```python
from build123d import *

# Parameters (mm, degrees)
SKETCH1_R              = 19
BOSS_EXTRUDE1_DEPTH    = 24
SKETCH2_R              = 13
CUT_EXTRUDE1_DEPTH     = 8
SKETCH3_R              = 6
CUT_EXTRUDE2_DEPTH     = 32.272991542
SKETCH4_R              = 12.5
CUT_EXTRUDE3_DEPTH     = 8
SKETCH5_W              = 22
SKETCH5_H              = 22
CUT_EXTRUDE4_DEPTH     = 8
CUT_EXTRUDE5_START     = 12
CUT_EXTRUDE5_OUTLINE_R = 6
CUT_EXTRUDE5_DEPTH     = 7.000000101
SKETCH6_R              = 1.5
CUT_EXTRUDE6_DEPTH     = 32.272991715
SKETCH7_R              = 1.5
CUT_EXTRUDE7_DEPTH     = 24


# Read off the part's stored shape, not the designer's step: Cut-Extrude5
with BuildPart() as part:
    # Sketch1 → Boss-Extrude1 (new body)
    with BuildSketch(Plane(origin=(0, 0, 0), x_dir=(1, 0, 0), z_dir=(0, 1, 0))):
        with Locations(Location((0, 0, 0), (0, 0, 270))):
            Circle(SKETCH1_R)
    extrude(amount=BOSS_EXTRUDE1_DEPTH)

    # Sketch2 → Cut-Extrude1 (cut)
    with BuildSketch(Plane(origin=(0, 24, 0), x_dir=(1, 0, 0), z_dir=(0, 1, 0))):
        with Locations(Location((0, 0, 0), (0, 0, 270))):
            Circle(SKETCH2_R)
    extrude(amount=-CUT_EXTRUDE1_DEPTH, mode=Mode.SUBTRACT)

    # Sketch3 → Cut-Extrude2 (cut, through all)
    with BuildSketch(Plane(origin=(0, 16, 0), x_dir=(1, 0, 0), z_dir=(0, 1, 0))):
        with Locations(Location((0, 0, 0), (0, 0, 270))):
            Circle(SKETCH3_R)
    extrude(amount=-CUT_EXTRUDE2_DEPTH, mode=Mode.SUBTRACT)

    # Sketch4 → Cut-Extrude3 (cut)
    with BuildSketch(Plane.XZ):
        with Locations(Location((0, 0, 0), (0, 0, 270))):
            Circle(SKETCH4_R)
    extrude(amount=-CUT_EXTRUDE3_DEPTH, mode=Mode.SUBTRACT)

    # Sketch5 → Cut-Extrude4 (cut)
    with BuildSketch(Plane.XZ):
        Rectangle(SKETCH5_W, SKETCH5_H)
    extrude(amount=-CUT_EXTRUDE4_DEPTH, mode=Mode.SUBTRACT)

    # Cut-Extrude5 outline → Cut-Extrude5 (cut)
    with BuildSketch(Plane.XY.offset(CUT_EXTRUDE5_START)):
        with Locations((-0.045844334, 12)):
            Circle(CUT_EXTRUDE5_OUTLINE_R)
    extrude(amount=CUT_EXTRUDE5_DEPTH, mode=Mode.SUBTRACT)

    # Sketch6 → Cut-Extrude6 (cut, through all)
    with BuildSketch(Plane(origin=(0, 16, 0), x_dir=(1, 0, 0), z_dir=(0, 1, 0))):
        with Locations(Location((-6.01040764, 6.01040764, 0), (0, 0, 270))):
            Circle(SKETCH6_R)
        with Locations(Location((6.01040764, -6.01040764, 0), (0, 0, 270))):
            Circle(SKETCH6_R)
    extrude(amount=-CUT_EXTRUDE6_DEPTH, mode=Mode.SUBTRACT)

    # Sketch7 → Cut-Extrude7 (cut)
    with BuildSketch(Plane(origin=(0, 24, 0), x_dir=(1, 0, 0), z_dir=(0, 1, 0))):
        with Locations(Location((11.313708499, -11.313708499, 0), (0, 0, 270))):
            Circle(SKETCH7_R)
        with Locations(Location((-11.313708499, -11.313708499, 0), (0, 0, 270))):
            Circle(SKETCH7_R)
        with Locations(Location((-11.313708499, 11.313708499, 0), (0, 0, 270))):
            Circle(SKETCH7_R)
        with Locations(Location((11.313708499, 11.313708499, 0), (0, 0, 270))):
            Circle(SKETCH7_R)
    extrude(amount=-CUT_EXTRUDE7_DEPTH, mode=Mode.SUBTRACT)


solid = part.part
```
Design review of the part built by this model. Coordinates are the model's own, in mm. A direction names the side the tool comes from. Round coordinates to 2 decimals unless told otherwise and drop trailing zeros. Order: outer loops, then holes, each group sorted by start corner. A loop starts at its lowest first (then second) coordinate and runs counter-clockwise, first axis right, second up. Notation, with made-up numbers: (-14.5, -3.75) - (11.5, -3.75) arc R15 cw to (11.5, 11.25) - close; hole circle Ø11 at (-38.75, -37). An arc over 180 degrees is marked (long way). Return JSON: item names as keys, results as strings.
Q1. Consider section B-B on z = 0. Write out the cut boundary in (x, y).
Computed values:
{"outline": "(-19, 0) - (-12.5, 0) - (-12.5, 8) - (-6, 8) - (-6, 16) - (-13, 16) - (-13, 24) - (-19, 24) - close; (6, 8) - (12.5, 8) - (12.5, 0) - (19, 0) - (19, 24) - (13, 24) - (13, 16) - (6, 16) - close"}
Q2. The part is to be moulded in two halves that separate along X. For faces 1 (the cylindrical face through (5.436, 12.056, 7.396)), 2 (the flat face through (-12.4, 0, 4)), 3 (the cylindrical face through (-11.56, 11.83, -15.08)), 4 (the cylindrical face through (12.58, 12.17, 12.12)), say which applies: pulls with the +X half, pulls with the -X half, needs draft (parallel to the pull), parting line crosses it, or undercut.
Computed values:
{"face 1": "undercut", "face 2": "needs draft", "face 3": "parting line crosses it", "face 4": "undercut"}
Q3. Machinability: for faces 5 (the flat face through (0, 12, 12)), 6 (the flat face through (8, 4, 11)), 7 (the flat face through (0.2, 16, -6.2)), which of the approach directions +Z, -Z, +X, -X, +Y, -Y give a long, thin tool a straight path to every point of the face, cutting with its end or side? Answer none if there is none.
Computed values:
{"face 5": "+Z", "face 6": "-Y", "face 7": "+Y"}
Q4. Consider section C-C on x = 1.5. Write out the cut boundary in (y, z), plus the area to 3 significant figures.
Computed values:
{"outline": "(0, -18.94) - (24, -18.94) - (24, -12.91) - (16, -12.91) - (16, -5.81) - (8, -5.81) - (8, -12.41) - (0, -12.41) - close; (0, 12.41) - (6.2, 12.41) - (6.2, 18.94) - (0, 18.94) - close; (8, 5.81) - (16, 5.81) - (16, 12) - (8, 12) - close; (17.8, 12.91) - (24, 12.91) - (24, 18.94) - (17.8, 18.94) - close", "area": "333 mm2"}
Q5. Wall thickness on L1, parallel to X at y = 20.5, z = -10; L2, parallel to X at y = 20, z = 0; L3, parallel to X at y = 10.25, z = -12.5: over which ranges is each line inside the solid? List them lowest first. Write a range as [from, to].
Computed values:
{"L1": "x = [-16.16, -12.04], [-10.59, -8.31], [8.31, 10.59], [12.04, 16.16]", "L2": "x = [-19, -13], [13, 19]", "L3": "x = [-14.31, -12.23], [-10.4, 10.4], [12.23, 14.31]"}
Q6. Consider section D-D on x = 7. Write out the cut boundary in (y, z), plus the area to 3 significant figures.
Computed values:
{"outline": "(0, -17.66) - (24, -17.66) - (24, -10.95) - (16, -10.95) - (16, 4.88) - (8, 4.88) - (8, -11) - (0, -11) - close; (0, 11) - (8, 11) - (8, 7.14) - (16, 7.14) - (16, 10.95) - (24, 10.95) - (24, 17.66) - (0, 17.66) - close", "area": "479 mm2"}
Q7. For pin 1 Ø1.2 at (y, z) = (4.5, -7) entering from +X; pin 2 Ø2.5 at (x, y) = (-0.5, 12) entering from +Z; pin 3 Ø1 at (x, y) = (-13.5, 19.5) entering from -Z, all flat-tipped, find the tip position at first contact; note any pin that passes through.
Computed values:
{"pin 1": "stops at x = 17.89", "pin 2": "stops at z = 12", "pin 3": "stops at z = -13.86"}
Q8. Consider section A-A on y = 1.75. Write out the cut boundary in (x, z), plus the area to 3 significant figures.
Computed values:
{"outline": "circle Ø38 at (0, 0); hole (-11, -9.85) arc R1.5 ccw (long way) to (-9.85, -11) - (-5.94, -11) arc R12.5 ccw to (5.94, -11) - (9.85, -11) arc R1.5 ccw (long way) to (11, -9.85) - (11, -5.94) arc R12.5 ccw to (11, 5.94) - (11, 9.85) arc R1.5 ccw (long way) to (9.85, 11) - (5.94, 11) arc R12.5 ccw to (-5.94, 11) - (-9.85, 11) arc R1.5 ccw (long way) to (-11, 9.85) - (-11, 5.94) arc R12.5 ccw to (-11, -5.94) - close", "area": "577 mm2"}
